```python
from build123d import *

# Parameters (mm, degrees)
F2_R     = 0.5
F3_DEPTH = 12.5
F4_W     = 2.789457
F4_H     = 0.8
F5_DEPTH = 13


with BuildPart() as f1:
    # F0 (on Front) → F1 (revolve)
    with BuildSketch(Plane.XZ):
        Polygon((1, 5), (0, 6), (0, 1.025), (25, 1.025), (25, 3), (23.267949, 2), (15.267949, 2), (15.267949, 3), (9.267949, 3), (9.267949, 4), (4.767949, 4), (4.767949, 5), align=None)
    revolve(axis=Axis((6.044726, 0, 0), (1, 0, 0)))

    # F2 (on Top) → F3 (cut, symmetric)
    with BuildSketch(Plane.XY):
        with Locations((3.057949, 0)):
            Circle(F2_R)
        with Locations((8.358715, 0)):
            Circle(F2_R)
        with Locations((13.456892, 0)):
            Circle(F2_R)
        with Locations((22.136655, 0)):
            Circle(F2_R)
    extrude(amount=F3_DEPTH, both=True, mode=Mode.SUBTRACT)

    # F4 (on face) → F5 (cut)
    with BuildSketch(Plane.YZ.offset(15.267949)):
        with Locations((-3.624397, 0)):
            Rectangle(F4_W, F4_H)
    extrude(amount=-F5_DEPTH, mode=Mode.SUBTRACT)


solid = f1.part
```
CAD build for the part. Positions are in the model's coordinates, mm. A direction names the side the tool comes from. Round coordinates to 2 decimals unless told otherwise and drop trailing zeros. Order: outer loops, then holes, each group sorted by start corner. A loop starts at its lowest first (then second) coordinate and runs counter-clockwise, first axis right, second up.
Item 1: Probe line 1 along X through (y, z) = (0, -1.4); line 2 along X through (y, z) = (0, -3.1); line 3 along X through (y, z) = (0, 2.55). List the from-to ranges inside material, lowest first.
Item 2: Mould opens along X. For faces 1 (the face through (2.56, 0.02, -2.92)), 2 (the face through (12.675, -1.016, -0.133)), 3 (the face through (9.268, 3, 1)) say: pulls with the +X half, pulls with the -X half, needs draft (parallel to the pull), parting line crosses it, or undercut.
Item 3: Saw through at A-A on z = 0. Write the cut outline in (x, y) (3 decimals), then the cut area to 3 significant figures.
Item 4: Saw through at C-C on x = 19.25. Write the cut outline in (y, z) (3 decimals), then the cut area to 3 significant figures.
Item 5: Tool access for faces 4 (the face through (12.957, 0.022, 1.933)), 5 (the face through (12, 3, 0)), 6 (the face through (7, -3, -0.4)), 7 (the face through (19.212, 0.766, 1.847)): list every direction of +Z, -Z, +X, -X, +Y, -Y with a clear straight run to the whole face (end or side of a thin tool).
Item 6: Saw through at B-B on y = 0. State how many separate pieces and enclosed holes the cut face has, then the cut area to 3 significant figures.
Item 7: Pin check, flat tips, straight feed: pin 1 (1.5 mm diameter, centred on x = 21.5, y = -1.5, fed in from -Z); pin 2 (1.6 mm diameter, centred on y = 0, z = 0, fed in from +X); pin 3 (3 mm diameter, centred on x = 15.5, y = -2.5, fed in from +Z); pin 4 (1.4 mm diameter, centred on x = 7.5, y = -3, fed in from +Z). Stop position of each tip, or through.
Reported:
1. line 1: x = 0 to 2.56, 3.56 to 7.86, 8.86 to 12.96, 13.96 to 21.64, 22.64 to 25
1. line 2: x = 0 to 2.56, 3.56 to 7.86, 8.86 to 9.27
1. line 3: x = 0 to 2.56, 3.56 to 7.86, 8.86 to 12.96, 13.96 to 15.27, 24.22 to 25
2. face 1: undercut
2. face 2: needs draft
2. face 3: pulls with the +X half
3. outline: (0, -6) - (1, -5) - (2.268, -5) - (2.268, -2.23) - (15.268, -2.23) - (15.268, -2) - (23.268, -2) - (25, -3) - (25, -1.025) - (0, -1.025) - close; (0, 1.025) - (25, 1.025) - (25, 3) - (23.268, 2) - (15.268, 2) - (15.268, 3) - (9.268, 3) - (9.268, 4) - (4.768, 4) - (4.768, 5) - (1, 5) - (0, 6) - close
3. area: 90.6 mm2
4. outline: circle Ø4 at (0, 0); hole circle Ø2.05 at (0, 0)
4. area: 9.27 mm2
5. face 4: +Z, -Z
5. face 5: +X
5. face 6: -Y
5. face 7: none
6. separate pieces: 10
6. enclosed holes: 0
6. area: 90.3 mm2
7. pin 1: stops at z = -1.85
7. pin 2: passes through
7. pin 3: stops at z = 2.82
7. pin 4: stops at z = 3.27
